Geometry: final body of the model. Coordinates: model frame, mm. Face numbers are marked on the shaded views. A direction names the side the tool comes from. Round coordinates to 2 decimals unless told otherwise and drop trailing zeros. Loops run counter-clockwise (first coordinate to the right, second up) from the corner with the lowest first, then second, coordinate; pieces in that order, holes last. Notation, with made-up numbers: (62.5, 86) -> (109.5, 86) arc R32 ccw to (109.5, 112) -> close; hole circle Ø11 at (-4.5, 44.5). An arc over 180 degrees is marked (long way). Answer in a Markdown table with one row per item.
```python
from build123d import *

# Parameters (mm, degrees)
BOSS_EXTRU_1_DEPTH      = 3
ESQUISSE2_R             = 1.5
ENL_V_MAT_EXTRU_1_DEPTH = 57.71860365
ESQUISSE3_R             = 3.5
BOSS_EXTRU_2_DEPTH      = 15
CONG_1_R                = 1
ESQUISSE4_W             = 30
ESQUISSE4_H             = 24.796786232
ENL_V_MAT_EXTRU_3_DEPTH = 1.5


with BuildPart() as part:
    # Esquisse1 → Boss.-Extru.1 (new body)
    with BuildSketch(Plane.XY):
        with BuildLine():
            Line((-18, 2), (0, 2))
            Line((0, 2), (0, 0))
            Line((0, 0), (-3, 0))
            ThreePointArc((-3, 0), (-0.866196648, -2.054890525), (2, -2.803628523))
            ThreePointArc((2, -2.803628523), (5.770289541, -2.076663576), (9, 0))
            Line((9, 0), (6, 0))
            Line((6, 0), (6, 2))
            Line((6, 2), (22, 2))
            Line((22, 2), (22, 42))
            Line((22, 42), (-18, 42))
            Line((-18, 42), (-38, 42))
            Line((-38, 42), (-38, -13))
            Line((-38, -13), (-18, -13))
            Line((-18, -13), (-18, 2))
        make_face()
    extrude(amount=BOSS_EXTRU_1_DEPTH)

    # Esquisse2 → Enlèv. mat.-Extru.1 (cut, through all)
    with BuildSketch(Plane.XY.offset(3)):
        with Locations((-16, 37.48988726)):
            Circle(ESQUISSE2_R)
        with Locations((-10.857142857, 37.48988726)):
            Circle(ESQUISSE2_R)
        with Locations((-5.714285714, 37.48988726)):
            Circle(ESQUISSE2_R)
        with Locations((-0.571428571, 37.48988726)):
            Circle(ESQUISSE2_R)
        with Locations((4.571428571, 37.48988726)):
            Circle(ESQUISSE2_R)
        with Locations((9.714285714, 37.48988726)):
            Circle(ESQUISSE2_R)
        with Locations((14.857142857, 37.48988726)):
            Circle(ESQUISSE2_R)
        with Locations((20, 37.48988726)):
            Circle(ESQUISSE2_R)
        with Locations((-10.857142857, 32.48988726)):
            Circle(ESQUISSE2_R)
        with Locations((-5.714285714, 32.48988726)):
            Circle(ESQUISSE2_R)
        with Locations((-0.571428571, 32.48988726)):
            Circle(ESQUISSE2_R)
        with Locations((4.571428571, 32.48988726)):
            Circle(ESQUISSE2_R)
        with Locations((9.714285714, 32.48988726)):
            Circle(ESQUISSE2_R)
        with Locations((14.857142857, 32.48988726)):
            Circle(ESQUISSE2_R)
        with Locations((-10.857142857, 27.48988726)):
            Circle(ESQUISSE2_R)
        with Locations((-5.714285714, 27.48988726)):
            Circle(ESQUISSE2_R)
        with Locations((-0.571428571, 27.48988726)):
            Circle(ESQUISSE2_R)
        with Locations((4.571428571, 27.48988726)):
            Circle(ESQUISSE2_R)
        with Locations((9.714285714, 27.48988726)):
            Circle(ESQUISSE2_R)
        with Locations((14.857142857, 27.48988726)):
            Circle(ESQUISSE2_R)
        with Locations((-10.857142857, 22.48988726)):
            Circle(ESQUISSE2_R)
        with Locations((-5.714285714, 22.48988726)):
            Circle(ESQUISSE2_R)
        with Locations((-0.571428571, 22.48988726)):
            Circle(ESQUISSE2_R)
        with Locations((4.571428571, 22.48988726)):
            Circle(ESQUISSE2_R)
        with Locations((9.714285714, 22.48988726)):
            Circle(ESQUISSE2_R)
        with Locations((14.857142857, 22.48988726)):
            Circle(ESQUISSE2_R)
        with Locations((-10.857142857, 17.48988726)):
            Circle(ESQUISSE2_R)
        with Locations((-5.714285714, 17.48988726)):
            Circle(ESQUISSE2_R)
        with Locations((-0.571428571, 17.48988726)):
            Circle(ESQUISSE2_R)
        with Locations((4.571428571, 17.48988726)):
            Circle(ESQUISSE2_R)
        with Locations((9.714285714, 17.48988726)):
            Circle(ESQUISSE2_R)
        with Locations((14.857142857, 17.48988726)):
            Circle(ESQUISSE2_R)
        with Locations((-10.857142857, 12.48988726)):
            Circle(ESQUISSE2_R)
        with Locations((-5.714285714, 12.48988726)):
            Circle(ESQUISSE2_R)
        with Locations((-0.571428571, 12.48988726)):
            Circle(ESQUISSE2_R)
        with Locations((4.571428571, 12.48988726)):
            Circle(ESQUISSE2_R)
        with Locations((9.714285714, 12.48988726)):
            Circle(ESQUISSE2_R)
        with Locations((14.857142857, 12.48988726)):
            Circle(ESQUISSE2_R)
        with Locations((-10.857142857, 7.48988726)):
            Circle(ESQUISSE2_R)
        with Locations((-5.714285714, 7.48988726)):
            Circle(ESQUISSE2_R)
        with Locations((-0.571428571, 7.48988726)):
            Circle(ESQUISSE2_R)
        with Locations((4.571428571, 7.48988726)):
            Circle(ESQUISSE2_R)
        with Locations((9.714285714, 7.48988726)):
            Circle(ESQUISSE2_R)
        with Locations((14.857142857, 7.48988726)):
            Circle(ESQUISSE2_R)
        with Locations((-16, 32.48988726)):
            Circle(ESQUISSE2_R)
        with Locations((-16, 27.48988726)):
            Circle(ESQUISSE2_R)
        with Locations((-16, 22.48988726)):
            Circle(ESQUISSE2_R)
        with Locations((-16, 17.48988726)):
            Circle(ESQUISSE2_R)
        with Locations((-16, 12.48988726)):
            Circle(ESQUISSE2_R)
        with Locations((-16, 7.48988726)):
            Circle(ESQUISSE2_R)
        with Locations((20, 32.48988726)):
            Circle(ESQUISSE2_R)
        with Locations((20, 27.48988726)):
            Circle(ESQUISSE2_R)
        with Locations((20, 22.48988726)):
            Circle(ESQUISSE2_R)
        with Locations((20, 17.48988726)):
            Circle(ESQUISSE2_R)
        with Locations((20, 12.48988726)):
            Circle(ESQUISSE2_R)
        with Locations((20, 7.48988726)):
            Circle(ESQUISSE2_R)
    extrude(amount=-ENL_V_MAT_EXTRU_1_DEPTH, mode=Mode.SUBTRACT)

    # Esquisse3 → Boss.-Extru.2 (add)
    with BuildSketch(Plane.XY.offset(3)):
        with Locations(Location((-30.5, 3.5, 0), (0, 0, 180))):
            Circle(ESQUISSE3_R)
    extrude(amount=BOSS_EXTRU_2_DEPTH)

    # Congé1
    cong_1_edges = [part.edges().sort_by_distance(p)[0] for p in [
        (-27, 3.5, 3),
    ]]
    fillet(cong_1_edges, radius=CONG_1_R)

    # Esquisse4 → Enlèv. mat.-Extru.3 (cut)
    with BuildSketch(Plane.XY):
        with Locations((2, 22)):
            Rectangle(ESQUISSE4_W, ESQUISSE4_H)
    extrude(amount=ENL_V_MAT_EXTRU_3_DEPTH, mode=Mode.SUBTRACT)


solid = part.part
```
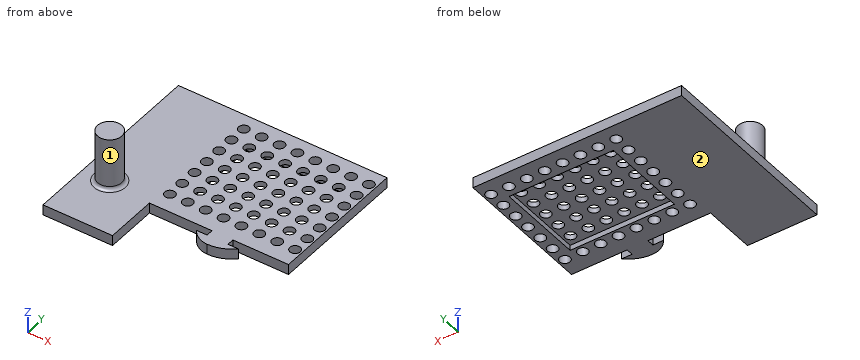
Item 1: Pin query (flat end, axial travel): pin 1 Ø3.5 at (x, y) = (-5.71, 17.49) entering from +Z; pin 2 Ø1.8 at (x, y) = (20, 37.49) entering from -Z; pin 3 Ø1.5 at (y, z) = (6, 9) entering from -X; pin 4 Ø5 at (x, y) = (-5.5, 17.5) entering from -Z. Return the tip coordinate at first contact, or that it passes through.
Answer:
| item | result |
|---|---|
| pin 1 | stops at z = 3 |
| pin 2 | passes through |
| pin 3 | stops at x = -33.53 |
| pin 4 | stops at z = 1.5 |
Item 2: Cut plane A-A (y = 3.5). Output: boundary loops of the cut face in (x, z).
Answer:
| item | result |
|---|---|
| outline | (-38, 0) -> (22, 0) -> (22, 3) -> (-26, 3) arc R1 cw to (-27, 4) -> (-27, 18) -> (-34, 18) -> (-34, 4) arc R1 cw to (-35, 3) -> (-38, 3) -> close |
Item 3: Cut plane D-D (z = 10.5). Output: boundary loops of the cut face in (x, y).
Answer:
| item | result |
|---|---|
| outline | circle Ø7 at (-30.5, 3.5) |
Item 4: Cut plane B-B (x = 20). Count the separate pieces of the cut face and the enclosed holes in it, then the cut area to 3 significant figures.
Answer:
| item | result |
|---|---|
| separate pieces | 8 |
| enclosed holes | 0 |
| area | 57.0 mm² |
Item 5: Cut plane C-C (x = -30.5). Output: boundary loops of the cut face in (y, z).
Answer:
| item | result |
|---|---|
| outline | (-13, 0) -> (42, 0) -> (42, 3) -> (8, 3) arc R1 cw to (7, 4) -> (7, 18) -> (0, 18) -> (0, 4) arc R1 cw to (-1, 3) -> (-13, 3) -> close |
Item 6: Reachability of the marked faces 1 and 2 from +Z, -Z, +X, -X, +Y, -Y: full face, straight path, thin tool, end or side. Return the list, or none.
Answer:
| item | result |
|---|---|
| face 1 | +Z |
| face 2 | -Z, +X, -X, +Y, -Y |
Item 7: Line query: probe 1 along Z at (x, y) = (-19.5, 12); probe 2 along Z at (x, y) = (7, 30.5); probe 3 along X at (y, z) = (5, 7.25). Output: solid intervals per line, ascending. Write a range as [from, to].
Answer:
| item | result |
|---|---|
| probe 1 | z = [0, 3] |
| probe 2 | z = [1.5, 3] |
| probe 3 | x = [-33.66, -27.34] |
